from build123d import *

# Parameters (mm, degrees)
F0_W     = 12
F0_H     = 10
F0_R     = 1.75
F1_DEPTH = 3.3
F2_SIZE  = 2
F3_R     = 3
F4_R     = 0.5
F5_DEPTH = 25


with BuildPart() as f1:
    # F0 (on Top) → F1 (new body)
    with BuildSketch(Plane.XY):
        Polygon((15, -15), (15, 15), (3, 15), (-15, 15), (-15, -15), align=None)
        with Locations((9, 20)):
            Rectangle(F0_W, F0_H)
        with Locations((9, 20)):
            Circle(F0_R, mode=Mode.SUBTRACT)
    extrude(amount=F1_DEPTH)

    # F2
    f2_edges = [f1.edges().sort_by_distance(p)[0] for p in [
        (3, 25, 1.65),
        (15, 25, 1.65),
    ]]
    chamfer(f2_edges, length=F2_SIZE)

    # F3
    f3_edges = [f1.edges().sort_by_distance(p)[0] for p in [
        (3, 15, 1.65),
    ]]
    fillet(f3_edges, radius=F3_R)

    # F4 (on face) → F5 (cut)
    with BuildSketch(Plane.XY.offset(3.3)):
        with Locations((-4.5, 0)):
            Circle(F4_R)
        with Locations((4.5, 0)):
            Circle(F4_R)
    extrude(amount=-F5_DEPTH, mode=Mode.SUBTRACT)


solid = f1.part
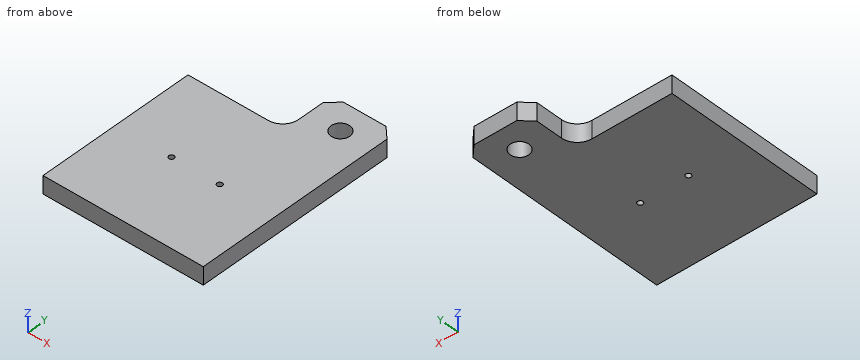
Could you check a few things on this model? Use its own coordinates, in mm. Give positions to 0.01 mm unless a question says otherwise; leave off trailing zeros. Order: outer loops, then holes, each group sorted by start corner. A loop starts at its lowest first (then second) coordinate and runs counter-clockwise, first axis right, second up.
Item 1: I'm going to push flat-ended pins straight in: pin 1 (3 mm diameter, centred on x = 9, y = 20, fed in from +Z); pin 2 (1.6 mm diameter, centred on x = -5, z = 1, fed in from +Y). Where does each tip first touch, or does it pass through?
Item 2: If we section it at A-A, the plane y = 20: Write out the boundary of the cut face in (x, z).
Item 3: If we section it at D-D, the plane x = -4.5: Write out the boundary of the cut face in (y, z).
Item 4: If we section it at B-B, the plane z = 2: Write out the boundary of the cut face in (x, y).
Item 5: If we section it at C-C, the plane y = 0: Write out the boundary of the cut face in (x, z).
Item 6: I need wall thicknesses on line 1 (Y direction, x = 9, z = 0.7); line 2 (Y direction, x = 4.5, z = 0.75); line 3 (Y direction, x = -9.5, z = 1.2). Which ranges of each line are inside material? Lowest first, please.
Values:
1. pin 1: passes through
1. pin 2: stops at y = 15
2. outline: (3, 0) - (7.25, 0) - (7.25, 3.3) - (3, 3.3) - close; (10.75, 0) - (15, 0) - (15, 3.3) - (10.75, 3.3) - close
3. outline: (-15, 0) - (-0.5, 0) - (-0.5, 3.3) - (-15, 3.3) - close; (0.5, 0) - (15, 0) - (15, 3.3) - (0.5, 3.3) - close
4. outline: (-15, -15) - (15, -15) - (15, 23) - (13, 25) - (5, 25) - (3, 23) - (3, 18) arc R3 cw to (0, 15) - (-15, 15) - close; hole circle Ø1 at (-4.5, 0); hole circle Ø1 at (4.5, 0); hole circle Ø3.5 at (9, 20)
5. outline: (-15, 0) - (-5, 0) - (-5, 3.3) - (-15, 3.3) - close; (-4, 0) - (4, 0) - (4, 3.3) - (-4, 3.3) - close; (5, 0) - (15, 0) - (15, 3.3) - (5, 3.3) - close
6. line 1: y = -15 to 18.25, 21.75 to 25
6. line 2: y = -15 to -0.5, 0.5 to 24.5
6. line 3: y = -15 to 15
